Study the drawing (mm; zero at the part's minimum x, y, z) and answer. A direction names the side the tool comes from. Give positions to 0.01 mm unless a question says otherwise; leave off trailing zeros. Write each loop counter-clockwise with the first axis right and the second up, starting at its lowest first coordinate (ties: lowest second). Pieces come first, ordered by that corner, then holes. Notation, with made-up numbers: (-32, -25.5) - (-26, -25.5) arc R17 cw to (-26, -19.5) - close; hole circle Ø5 at (-19.75, -30). An arc over 180 degrees is marked (long way). Answer as CSV lines item,"result".
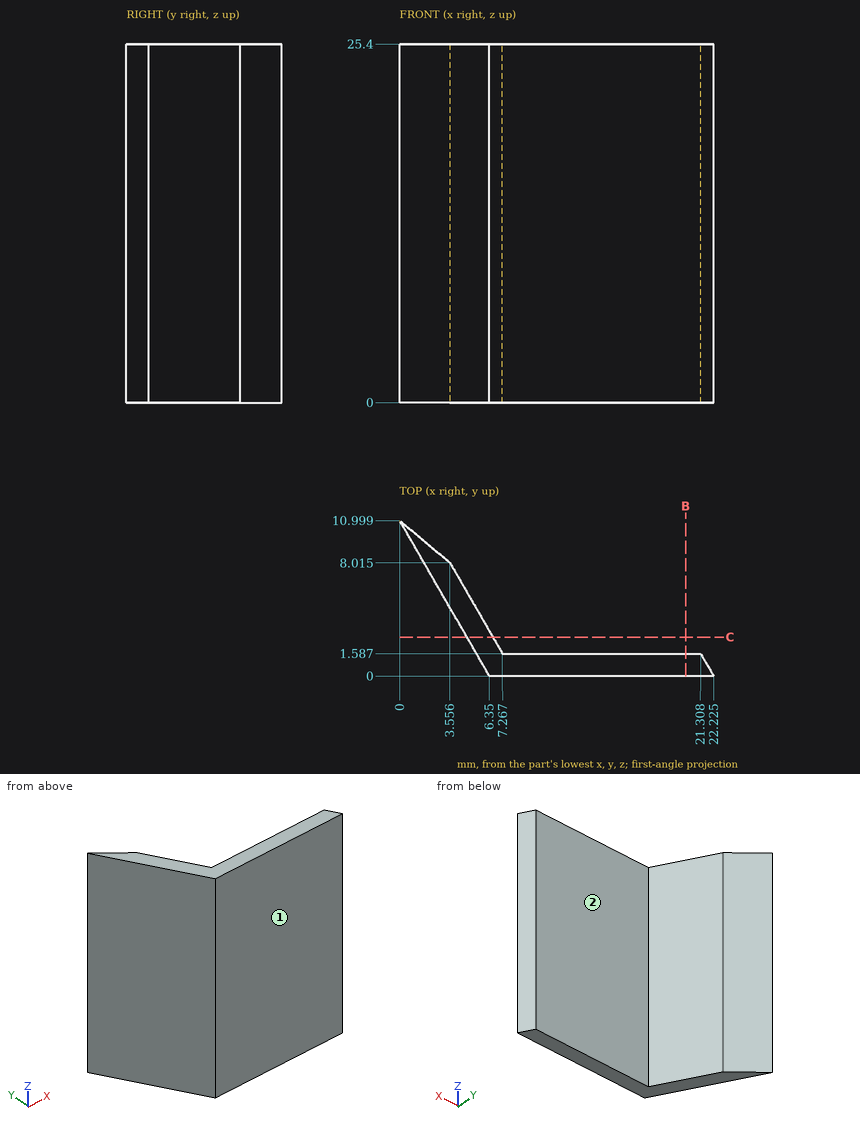
(1) Find the intervals of material crossed by L1, parallel to Y at x = 11.25, z = 24; L2, parallel to X at y = 7.25, z = 11 (1 decimal); L3, parallel to X at y = 2.5, z = 23.5 (1 decimal), in increasing order.
Worked out:
L1,"y = 0 to 1.59"
L2,"x = 2.2 to 4"
L3,"x = 4.9 to 6.7"
(2) A cutting plane is placed at B-B (x = 20.25). Write down the section's boundary in (y, z).
Worked out:
outline,"(0, 0) - (1.59, 0) - (1.59, 25.4) - (0, 25.4) - close"
(3) Each of these flat-tipped pins is pushed along its axis until it touches: P1, Ø6, axis at x = 5.5, z = 14.5, coming from the +Y side; P2, Ø1.5, axis at y = 6.5, z = 17, coming from the +X side; P3, Ø6, axis at y = 6, z = 5.5, coming from the +X side. Where does it stop, or does it pass through?
Worked out:
P1,"stops at y = 8.9"
P2,"stops at x = 4.86"
P3,"stops at x = 6.45"
(4) For the marked faces 1 and 2, determine the directions among +Z, -Z, +X, -X, +Y, -Y from which every point of the face is accessible in a straight line to the end or side of a thin tool.
Worked out:
face 1,"+Z, -Z, +X, -X, -Y"
face 2,"+Z, -Z, +X, +Y"
(5) A cutting plane is placed at C-C (y = 2.75). Write down the section's boundary in (x, z) (1 decimal).
Worked out:
outline,"(4.8, 0) - (6.6, 0) - (6.6, 25.4) - (4.8, 25.4) - close"
